Part model, mm, in its own coordinate system. Face numbers are marked on the shaded views. Coordinates: 2 decimals unless noted, no trailing zeros. Order: outer loops, then holes, each group sorted by start corner. A loop starts at its lowest first (then second) coordinate and runs counter-clockwise, first axis right, second up.
```python
from build123d import *

# Parameters (mm, degrees)
F0_R     = 7.5
F1_DEPTH = 10
F0_W     = 99
F0_H     = 88
F0_R_2   = 4.75
F2_DEPTH = 15
F3_R     = 25
F3_R_2   = 7.5
F4_DEPTH = 3


with BuildPart() as f1:
    # F0 (on Top) → F1 (new body)
    with BuildSketch(Plane.XY):
        Circle(F0_R)
    extrude(amount=F1_DEPTH)

    # F0 (on Top) → F2 (join)
    with BuildSketch(Plane.XY):
        Rectangle(F0_W, F0_H)
        with Locations((-31, -30)):
            Circle(F0_R_2, mode=Mode.SUBTRACT)
        with Locations((31, -30)):
            Circle(F0_R_2, mode=Mode.SUBTRACT)
        with Locations((-31, 30)):
            Circle(F0_R_2, mode=Mode.SUBTRACT)
        Circle(F0_R, mode=Mode.SUBTRACT)
        with Locations((31, 30)):
            Circle(F0_R_2, mode=Mode.SUBTRACT)
    extrude(amount=F2_DEPTH)

    # F3 (on face) + F0 (on Top) → F4 (cut)
    with BuildSketch(Plane.XY):
        Circle(F3_R)
        Circle(F3_R_2, mode=Mode.SUBTRACT)
    with BuildSketch(Plane.XY):
        Circle(F0_R)
    extrude(amount=F4_DEPTH, mode=Mode.SUBTRACT)


solid = f1.part
```
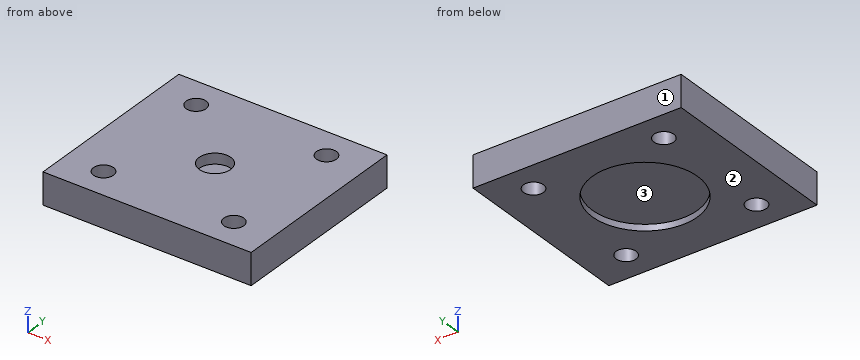
(1) Slice it at A-A, the plane x = 31. Give the cut face in (y, z), then the cut area to 4 significant figures.
(2) Probe line 1 (X direction, y = 29.5, z = 1.5); line 2 (Y direction, x = -31, z = 3.75); line 3 (Y direction, x = 0, z = 0.9). List the from-to ranges inside material, lowest first.
(3) Slice it at B-B, the plane z = 13.25. Give the cut face in (x, y).
(4) Drop flat-ended pins along their axis: pin 1 (6 mm diameter, centred on x = 5.5, y = -16, fed in from -Z); pin 2 (12.5 mm diameter, centred on x = 31, y = -30, fed in from -Z); pin 3 (4.5 mm diameter, centred on x = 3.5, y = 1, fed in from +Z); pin 4 (8.5 mm diameter, centred on x = 31, y = 30, fed in from -Z). Give the stop position or say it passes through.
(5) Slice it at D-D, the plane x = 0. Give the cut face in (y, z).
(6) Slice it at C-C, the plane y = 0. Give the cut face in (x, z).
(7) Pull direction Y, two halves, no side cores. Call the marked faces 1, 2 and 3: +Y half, -Y half, draft (parallel to the pull), parting line (faces both ways), or undercut.
Here are the results:
1. outline: (-44, 0) - (-34.75, 0) - (-34.75, 15) - (-44, 15) - close; (-25.25, 0) - (25.25, 0) - (25.25, 15) - (-25.25, 15) - close; (34.75, 0) - (44, 0) - (44, 15) - (34.75, 15) - close
1. area: 1,035 mm2
2. line 1: x = -49.5 to -35.72, -26.28 to 26.28, 35.72 to 49.5
2. line 2: y = -44 to -34.75, -25.25 to 25.25, 34.75 to 44
2. line 3: y = -44 to -25, 25 to 44
3. outline: (-49.5, -44) - (49.5, -44) - (49.5, 44) - (-49.5, 44) - close; hole circle Ø9.5 at (-31, -30); hole circle Ø9.5 at (-31, 30); hole circle Ø15 at (0, 0); hole circle Ø9.5 at (31, -30); hole circle Ø9.5 at (31, 30)
4. pin 1: stops at z = 3
4. pin 2: stops at z = 0
4. pin 3: stops at z = 10
4. pin 4: passes through
5. outline: (-44, 0) - (-25, 0) - (-25, 3) - (25, 3) - (25, 0) - (44, 0) - (44, 15) - (7.5, 15) - (7.5, 10) - (-7.5, 10) - (-7.5, 15) - (-44, 15) - close
6. outline: (-49.5, 0) - (-25, 0) - (-25, 3) - (25, 3) - (25, 0) - (49.5, 0) - (49.5, 15) - (7.5, 15) - (7.5, 10) - (-7.5, 10) - (-7.5, 15) - (-49.5, 15) - close
7. face 1: +Y half
7. face 2: draft
7. face 3: undercut
